```python
from build123d import *

# Parameters (mm, degrees)
SKETCH1_R           = 5.15
SKETCH1_R_2         = 7.55
SKETCH1_R_3         = 5.05
SKETCH1_R_4         = 1.5
SKETCH1_R_5         = 2.165
BOSS_EXTRUDE1_DEPTH = 12


with BuildPart() as part:
    # Sketch1 → Boss-Extrude1 (new body)
    with BuildSketch(Plane(origin=(0, 0, 0), x_dir=(1, 0, 0), z_dir=(0, 1, 0))):
        with BuildLine():
            Line((-2.036490016, 62.232628927), (-23.679041405, 66.734453302))
            ThreePointArc((-23.679041405, 66.734453302), (-38.872266056, 60.051931597), (-37.504850395, 43.510458082))
            Line((-37.504850395, 43.510458082), (-28.95403297, 33.398266841))
            ThreePointArc((-28.95403297, 33.398266841), (-27.199588127, 30.379378664), (-26.59, 26.941332001))
            Line((-26.59, 26.941332001), (-26.59, 4.037047599))
            ThreePointArc((-26.59, 4.037047599), (-27.829524982, -0.785200575), (-31.240815491, -4.411989333))
            Line((-31.240815491, -4.411989333), (-44.914180747, -13.06875746))
            ThreePointArc((-44.914180747, -13.06875746), (-48.938899729, -30.983792167), (-31.023865021, -35.008511149))
            Line((-31.023865021, -35.008511149), (-22.386088755, -29.539833551))
            ThreePointArc((-22.386088755, -29.539833551), (-20.83471499, -28.738106539), (-19.167525971, -28.21848405))
            Line((-19.167525971, -28.21848405), (-2.130621725, -24.503257579))
            ThreePointArc((-2.130621725, -24.503257579), (0, -24.273644012), (2.130621725, -24.503257579))
            Line((2.130621725, -24.503257579), (19.167525971, -28.21848405))
            ThreePointArc((19.167525971, -28.21848405), (20.83471499, -28.738106539), (22.386088755, -29.539833551))
            Line((22.386088755, -29.539833551), (31.023865021, -35.008511149))
            ThreePointArc((31.023865021, -35.008511149), (48.938899729, -30.983792167), (44.914180747, -13.06875746))
            Line((44.914180747, -13.06875746), (31.240815491, -4.411989333))
            ThreePointArc((31.240815491, -4.411989333), (27.829524982, -0.785200575), (26.59, 4.037047599))
            Line((26.59, 4.037047599), (26.59, 26.941332001))
            ThreePointArc((26.59, 26.941332001), (27.199588127, 30.379378664), (28.95403297, 33.398266841))
            Line((28.95403297, 33.398266841), (37.504850395, 43.510458082))
            ThreePointArc((37.504850395, 43.510458082), (38.872266056, 60.051931597), (23.679041405, 66.734453302))
            Line((23.679041405, 66.734453302), (2.036490016, 62.232628927))
            ThreePointArc((2.036490016, 62.232628927), (0, 62.023068571), (-2.036490016, 62.232628927))
        make_face()
        Circle(SKETCH1_R, mode=Mode.SUBTRACT)
        with Locations((-31.59, -20)):
            Circle(SKETCH1_R_2, mode=Mode.SUBTRACT)
        with Locations((-26.59, 52.74)):
            Circle(SKETCH1_R_3, mode=Mode.SUBTRACT)
        with Locations((-26.59, 60.99)):
            Circle(SKETCH1_R_4, mode=Mode.SUBTRACT)
        with Locations((-18.34, 52.74)):
            Circle(SKETCH1_R_4, mode=Mode.SUBTRACT)
        with Locations((-26.59, 44.49)):
            Circle(SKETCH1_R_4, mode=Mode.SUBTRACT)
        with Locations((-34.84, 52.74)):
            Circle(SKETCH1_R_4, mode=Mode.SUBTRACT)
        with Locations((-42.286480756, -26.772067589)):
            Circle(SKETCH1_R_5, mode=Mode.SUBTRACT)
        with Locations((-20.893519244, -13.227932411)):
            Circle(SKETCH1_R_5, mode=Mode.SUBTRACT)
        with Locations((20.893519244, -13.227932411)):
            Circle(SKETCH1_R_5, mode=Mode.SUBTRACT)
        with Locations((42.286480756, -26.772067589)):
            Circle(SKETCH1_R_5, mode=Mode.SUBTRACT)
        with Locations((34.84, 52.74)):
            Circle(SKETCH1_R_4, mode=Mode.SUBTRACT)
        with Locations((26.59, 44.49)):
            Circle(SKETCH1_R_4, mode=Mode.SUBTRACT)
        with Locations((18.34, 52.74)):
            Circle(SKETCH1_R_4, mode=Mode.SUBTRACT)
        with Locations((26.59, 60.99)):
            Circle(SKETCH1_R_4, mode=Mode.SUBTRACT)
        with Locations((26.59, 52.74)):
            Circle(SKETCH1_R_3, mode=Mode.SUBTRACT)
        with Locations((31.59, -20)):
            Circle(SKETCH1_R_2, mode=Mode.SUBTRACT)
    extrude(amount=BOSS_EXTRUDE1_DEPTH)


solid = part.part
```
Read the model definition and answer for the solid it produces. Units are mm, in the model's axes. A direction names the side the tool comes from. Round coordinates to 2 decimals unless told otherwise and drop trailing zeros. Write each loop counter-clockwise with the first axis right and the second up, starting at its lowest first coordinate (ties: lowest second). Pieces come first, ordered by that corner, then holes. Notation, with made-up numbers: (2.25, -39.75) -> (23.25, -39.75) arc R18 ccw to (23.25, -21.75) -> close; hole circle Ø5 at (85, 88). An arc over 180 degrees is marked (long way). Answer in a Markdown table with one row per item. Add a question column.
1) Which of the six approach directions +Z, -Z, +X, -X, +Y, -Y give full straight-line access (tool end or side, diameter ignored) to faces 5 (the face through (-27.22, 5.92, -30.43)), 6 (the face through (10.53, 5.916, 26.335)), 7 (the face through (-25.204, 5.916, -43.915)), 8 (the face through (27.18, 5.92, -30.33))?
2) Find section C-C, the plane y = 8.75. State how many separate pieces and enclosed holes the cut face has, and give its area (3 significant figures).
3) Find section B-B, the plane z = 20. Determine the outline of the cut face in (x, y).
4) Determine the mould class of faces 1 (the face through (-20.86, 5.92, 28.75)), 2 (the face through (0.029, 5.916, -62.023)), 3 (the face through (-27.796, 5.916, 0.723)), 4 (the face through (48.8, 5.9, 31.2)) for opening direction Z: pulls with the +Z half, pulls with the -Z half, needs draft (parallel to the pull), parting line crosses it, or undercut.
5) Find section A-A, the plane x = 34.84. Determine the outline of the cut face in (y, z).
6) Find section D-D, the plane z = -49.5. Determine the outline of the cut face in (x, y).
7) Given P1, Ø2.5, axis at x = 26.59, z = -44.49, coming from the +Y side; P2, Ø3.5, axis at y = 9, z = -16.5, coming from the -X side; P3, Ø4, axis at y = 7, z = -55.5, coming from the -X side; P4, Ø1, axis at y = 2, z = -42, coming from the -X side, each flat-ended and moving along its own axis, determine where each tip first touches the part or whether it passes through.
8) Consider line 1 (Z direction, x = -19.5, y = 5.5); line 2 (Z direction, x = 34.84, y = 9.75); line 3 (X direction, y = 2, z = 16.5). Determine where each line is inside the solid, lowest interval first.
Findings below:
| question | item | result |
|---|---|---|
| 1 | face 5 | -X, +Y, -Y |
| 1 | face 6 | +Z, +Y, -Y |
| 1 | face 7 | +Y, -Y |
| 1 | face 8 | +X, +Y, -Y |
| 2 | separate pieces | 1 |
| 2 | enclosed holes | 17 |
| 2 | area | 6,110 mm² |
| 3 | outline | (-50.31, 0) -> (-39.14, 0) -> (-39.14, 12) -> (-50.31, 12) -> close; (-24.04, 0) -> (24.04, 0) -> (24.04, 12) -> (-24.04, 12) -> close; (39.14, 0) -> (50.31, 0) -> (50.31, 12) -> (39.14, 12) -> close |
| 4 | face 1 | pulls with the +Z half |
| 4 | face 2 | pulls with the -Z half |
| 4 | face 3 | undercut |
| 4 | face 4 | parting line crosses it |
| 5 | outline | (0, -64.41) -> (12, -64.41) -> (12, -54.24) -> (0, -54.24) -> close; (0, -51.24) -> (12, -51.24) -> (12, -40.36) -> (0, -40.36) -> close; (0, 6.69) -> (12, 6.69) -> (12, 13.19) -> (0, 13.19) -> close; (0, 26.81) -> (12, 26.81) -> (12, 36.64) -> (0, 36.64) -> close |
| 6 | outline | (-40.51, 0) -> (-30.46, 0) -> (-30.46, 12) -> (-40.51, 12) -> close; (-22.72, 0) -> (22.72, 0) -> (22.72, 12) -> (-22.72, 12) -> close; (30.46, 0) -> (40.51, 0) -> (40.51, 12) -> (30.46, 12) -> close |
| 7 | P1 | through |
| 7 | P2 | x = -26.59 |
| 7 | P3 | x = -40.86 |
| 7 | P4 | x = -36.65 |
| 8 | line 1 | -65.87 to -53.69, -51.79 to 11.57, 14.88 to 28.3 |
| 8 | line 2 | -64.41 to -54.24, -51.24 to -40.36, 6.69 to 13.19, 26.81 to 36.64 |
| 8 | line 3 | -48.54 to -38.28, -24.9 to 24.9, 38.28 to 48.54 |
